Build history of the part. All positions in model axes, mm. Face numbers are marked on the shaded views. A direction names the side the tool comes from. Give positions to 0.01 mm unless a question says otherwise; leave off trailing zeros. Order: outer loops, then holes, each group sorted by start corner. A loop starts at its lowest first (then second) coordinate and runs counter-clockwise, first axis right, second up. Notation, with made-up numbers: (37.5, -1.5) -> (90.5, -1.5) arc R23 ccw to (90.5, 19.5) -> close; hole circle Ø1 at (-35, 83.5). An arc over 180 degrees is marked (long way). One line per question, with ' | ' between items. Start each with the question number.
(1) Which spindle directions (+Z, -Z, +X, -X, +Y, -Y) get a long thin tool onto all of the face, cutting with end or side? Do the marked faces 1, 2, 3 and 4. Say none if no direction does.
(2) Pin check, flat tips, straight feed: pin 1 Ø8 at (y, z) = (27.5, 5.5) entering from -X; pin 2 Ø8 at (x, y) = (7, 17.5) entering from +Z; pin 3 Ø2 at (x, z) = (25, 51.5) entering from +Y. Stop position of each tip, or through.
(3) Cut at A-A (z = 67.5). Give the cut face in (x, y).
(4) Cut at B-B (y = 7). Give the cut face in (x, z).
(5) Drill centre lines: L1, parallel to X at y = -5, z = 72.5; L2, parallel to Z at x = 11.5, y = 5.5; L3, parallel to Y at x = -26, z = 53. Where is each one in solid material? Low to high. Write a range as from..to.
(6) Pull direction X, two halves, no side cores. Call the marked faces 5, 6, 7 and 8: +X half, -X half, draft (parallel to the pull), parting line (faces both ways), or undercut.
(7) Cut at C-C (x = 20.5). Give the cut face in (y, z).
(8) Cut at D-D (y = 0). Give the cut face in (x, z).
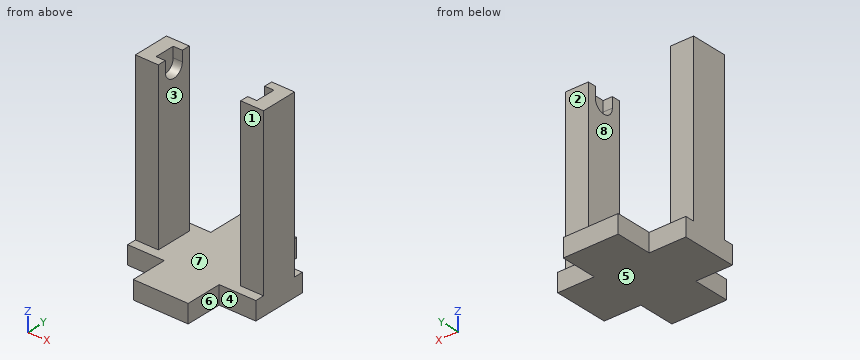
from build123d import *

# Parameters (mm, degrees)
F0_W     = 20
F0_H     = 30
F0_W_2   = 30
F0_H_2   = 20
F1_DEPTH = 10
F2_W     = 12.5
F2_H     = 20
F3_DEPTH = 100
F5_DEPTH = 27.5


with BuildPart() as f1:
    # F0 (on Top) → F1 (new body)
    with BuildSketch(Plane.XY):
        with Locations((25, 0)):
            Rectangle(F0_W, F0_H)
        with Locations((0, -25)):
            Rectangle(F0_W_2, F0_H_2)
        Rectangle(F0_W_2, F0_H)
        with Locations((-25, 0)):
            Rectangle(F0_W, F0_H)
        with Locations((0, 25)):
            Rectangle(F0_W_2, F0_H_2)
    extrude(amount=F1_DEPTH)

    # F2 (on Top) → F3 (join)
    with BuildSketch(Plane.XY):
        with Locations((-28.75, 0)):
            Rectangle(F2_W, F2_H)
        with Locations((28.75, 0)):
            Rectangle(F2_W, F2_H)
    extrude(amount=F3_DEPTH)

    # F4 (on Right) → F5 (cut, symmetric)
    with BuildSketch(Plane.YZ):
        with BuildLine():
            Line((-5.5, 100), (-5.5, 94.3625420332))
            ThreePointArc((-5.5, 94.3625420332), (0, 88.8625420332), (5.5, 94.3625420332))
            Line((5.5, 94.3625420332), (5.5, 100))
            Line((5.5, 100), (-5.5, 100))
        make_face()
    extrude(amount=F5_DEPTH, both=True, mode=Mode.SUBTRACT)


solid = f1.part
Result set:
1) face 1: +Z, +X, -X, -Y | face 2: +Z, +X, -X, +Y | face 3: +Z, +Y, -Y | face 4: +Z, -Z, +X, -Y
2) pin 1: stops at x = -15 | pin 2: stops at z = 10 | pin 3: stops at y = 10
3) outline: (-35, -10) -> (-22.5, -10) -> (-22.5, 10) -> (-35, 10) -> close; (22.5, -10) -> (35, -10) -> (35, 10) -> (22.5, 10) -> close
4) outline: (-35, 0) -> (35, 0) -> (35, 100) -> (22.5, 100) -> (22.5, 10) -> (-22.5, 10) -> (-22.5, 100) -> (-35, 100) -> close
5) L1: x = -35..-22.5, 22.5..35 | L2: z = 0..10 | L3: y = -10..10
6) face 5: draft | face 6: +X half | face 7: undercut | face 8: undercut
7) outline: (-15, 0) -> (15, 0) -> (15, 10) -> (-15, 10) -> close
8) outline: (-35, 0) -> (35, 0) -> (35, 100) -> (27.5, 100) -> (27.5, 88.86) -> (22.5, 88.86) -> (22.5, 10) -> (-22.5, 10) -> (-22.5, 88.86) -> (-27.5, 88.86) -> (-27.5, 100) -> (-35, 100) -> close
